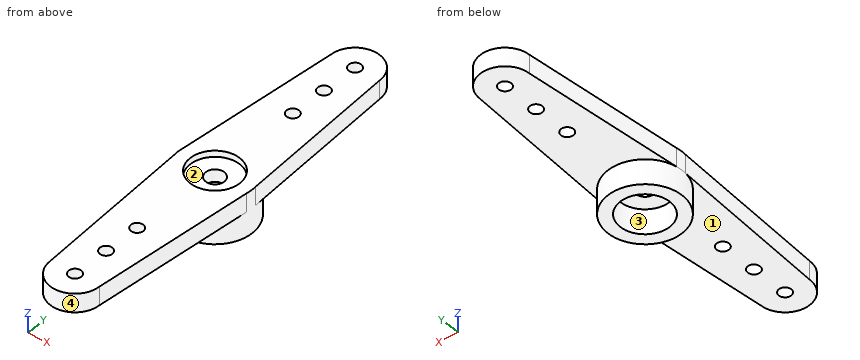
```python
from build123d import *

# Parameters (mm, degrees)
BOSS_EXTRU_2_DEPTH         = 1.5
ESQUISSE2_R                = 3
ESQUISSE2_R_2              = 2
BOSS_EXTRU_3_DEPTH         = 2
ESQUISSE3_R                = 0.75
ENL_V_MAT_EXTRU_1_DEPTH    = 2
ESQUISSE4_R                = 2
ENL_V_MAT_EXTRU_2_DEPTH    = 0.5
ESQUISSE5_R                = 0.5
ENL_V_MAT_EXTRU_3_DEPTH    = 4.5
R_P_TITION_LIN_AIRE1_COUNT = 3
R_P_TITION_LIN_AIRE1_PITCH = 3
SYM_TRIE1_COPY_1_SKETCH_R  = 0.5
SYM_TRIE1_COPY_1_DEPTH     = 4.5
SYM_TRIE1_COPY_2_SKETCH_R  = 0.5
SYM_TRIE1_COPY_2_DEPTH     = 4.5


with BuildPart() as part:
    # Esquisse1 → Boss.-Extru.2 (new body)
    with BuildSketch(Plane.XY):
        with BuildLine():
            Line((2, 13.5), (2.967257844, 0.4420191))
            ThreePointArc((2.967257844, 0.4420191), (3, 0), (2.967257844, -0.4420191))
            Line((2.967257844, -0.4420191), (2, -13.5))
            ThreePointArc((2, -13.5), (0, -15.5), (-2, -13.5))
            Line((-2, -13.5), (-2.967257844, -0.4420191))
            ThreePointArc((-2.967257844, -0.4420191), (-3, 0), (-2.967257844, 0.4420191))
            Line((-2.967257844, 0.4420191), (-2, 13.5))
            ThreePointArc((-2, 13.5), (0, 15.5), (2, 13.5))
        make_face()
    extrude(amount=BOSS_EXTRU_2_DEPTH)

    # Esquisse2 → Boss.-Extru.3 (add)
    with BuildSketch(Plane(origin=(0, 0, 0), x_dir=(-1, 0, 0), z_dir=(0, 0, -1))):
        Circle(ESQUISSE2_R)
        Circle(ESQUISSE2_R_2, mode=Mode.SUBTRACT)
    extrude(amount=BOSS_EXTRU_3_DEPTH)

    # Esquisse3 → Enlèv. mat.-Extru.1 (cut)
    with BuildSketch(Plane(origin=(0, 0, 0), x_dir=(-1, 0, 0), z_dir=(0, 0, -1))):
        Circle(ESQUISSE3_R)
    extrude(amount=-ENL_V_MAT_EXTRU_1_DEPTH, mode=Mode.SUBTRACT)

    # Esquisse4 → Enlèv. mat.-Extru.2 (cut)
    with BuildSketch(Plane.XY.offset(1.5)):
        Circle(ESQUISSE4_R)
    extrude(amount=-ENL_V_MAT_EXTRU_2_DEPTH, mode=Mode.SUBTRACT)

    # Esquisse5 → Enlèv. mat.-Extru.3 (cut, through all)
    with BuildSketch(Plane.XY.offset(1.5)):
        with Locations((0, 13.5)):
            Circle(ESQUISSE5_R)
    enl_v_mat_extru_3 = extrude(amount=-ENL_V_MAT_EXTRU_3_DEPTH, mode=Mode.SUBTRACT)

    # Répétition linéaire1: Enlèv. mat.-Extru.3 ×3
    with Locations(*[(0, -i * R_P_TITION_LIN_AIRE1_PITCH, 0) for i in range(1, R_P_TITION_LIN_AIRE1_COUNT)]):
        add(enl_v_mat_extru_3, mode=Mode.SUBTRACT)

    # Symétrie1: Enlèv. mat.-Extru.3 across plane
    add(enl_v_mat_extru_3.mirror(Plane.ZX), mode=Mode.SUBTRACT)

    # Symétrie1 copy 1 sketch → Symétrie1 copy 1 (cut, through all)
    with BuildSketch(Plane(origin=(0, 3, 1.5), x_dir=(1, 0, 0), z_dir=(0, 0, 1))):
        with Locations((0, -13.5)):
            Circle(SYM_TRIE1_COPY_1_SKETCH_R)
    extrude(amount=-SYM_TRIE1_COPY_1_DEPTH, mode=Mode.SUBTRACT)

    # Symétrie1 copy 2 sketch → Symétrie1 copy 2 (cut, through all)
    with BuildSketch(Plane(origin=(0, 6, 1.5), x_dir=(1, 0, 0), z_dir=(0, 0, 1))):
        with Locations((0, -13.5)):
            Circle(SYM_TRIE1_COPY_2_SKETCH_R)
    extrude(amount=-SYM_TRIE1_COPY_2_DEPTH, mode=Mode.SUBTRACT)


solid = part.part
```
Check sheet for the modelled part. Datum: model origin and axes. Units: mm. Face numbers are marked on the shaded views. Coordinates: 2 decimals unless noted, no trailing zeros. Loops run counter-clockwise (first coordinate to the right, second up) from the corner with the lowest first, then second, coordinate; pieces in that order, holes last. Notation, with made-up numbers: M 75,40 L 131,40 A22 cw 131,72 Z; hole C 87.25,66.25 d8. An arc over 180 degrees is marked long. Answer as a JSON object with one key per item and string values.
1. Sectioned sample at C-C on x = 0. Count the separate pieces of the cut face and the enclosed holes in it, and give its area (3 significant figures).
Outcome:
{"separate pieces": "8", "enclosed holes": "0", "area": "38.0 mm²"}
2. Release check for a two-part mould opening along X. For the marked faces 1, 2, 3 and 4 record: pulls with the +X half, pulls with the -X half, needs draft (parallel to the pull), parting line crosses it, or undercut.
Outcome:
{"face 1": "needs draft", "face 2": "undercut", "face 3": "undercut", "face 4": "parting line crosses it"}
3. Sectioned sample at B-B on y = 7.5. Record the cut outline in (x, z), and give its area (3 significant figures).
Outcome:
{"outline": "M -2.44,0 L -0.5,0 L -0.5,1.5 L -2.44,1.5 Z; M 0.5,0 L 2.44,0 L 2.44,1.5 L 0.5,1.5 Z", "area": "5.83 mm²"}
4. Sectioned sample at A-A on z = 0.4. Record the cut outline in (x, y), and give its area (3 significant figures).
Outcome:
{"outline": "M -2.97,-0.44 L -2,-13.5 A2 ccw 2,-13.5 L 2.97,-0.44 A3 ccw 2.97,0.44 L 2,13.5 A2 ccw -2,13.5 L -2.97,0.44 A3 ccw Z; hole C 0,0 d1.5; hole C 0,-13.5 d1; hole C 0,-10.5 d1; hole C 0,-7.5 d1; hole C 0,7.5 d1; hole C 0,10.5 d1; hole C 0,13.5 d1", "area": "141 mm²"}
5. Scan lines: L1, parallel to Z at x = 1.5, y = -4.5; L2, parallel to X at y = 1, z = -0.85; L3, parallel to X at y = 1.5, z = 1.2. Record each from-to range of solid material in increasing order. Write a range as from..to.
Outcome:
{"L1": "0..1.5", "L2": "-2.83..-1.73, 1.73..2.83", "L3": "-2.89..-1.32, 1.32..2.89"}
6. Depth check by flat-ended pin: P1, Ø1.2, axis at x = -0.5, y = 0, coming from the -Z side; P2, Ø1, axis at x = -1, z = -1.5, coming from the +Y side; P3, Ø1.4, axis at x = 0, y = 0, coming from the -Z side. Enter the tip coordinate at first touch or a pass-through.
Outcome:
{"P1": "z = 0", "P2": "y = 2.96", "P3": "through"}
7. Sectioned sample at D-D on z = -1.7. Record the cut outline in (x, y), and give its area (3 significant figures).
Outcome:
{"outline": "C 0,0 d6; hole C 0,0 d4", "area": "15.7 mm²"}
